Geometry: final body of the model. Coordinates: model frame, mm. Give positions to 0.01 mm unless a question says otherwise; leave off trailing zeros. Loops run counter-clockwise (first coordinate to the right, second up) from the corner with the lowest first, then second, coordinate; pieces in that order, holes last. Notation, with made-up numbers: M 2.5,35 L 34.5,35 A16 ccw 34.5,52 Z; hole C 31,-2.5 d10. An arc over 180 degrees is marked long. One line per question, with ' | ' between items. Start each with the question number.
from build123d import *

# Parameters (mm, degrees)
F0_W        = 105
F0_H        = 20.7723644742
F1_DEPTH    = 3
F2_T1_DEPTH = 58


# Not quite as in the source:
# - a fillet or chamfer that OpenCascade refuses, or shapes differently, is made with other operations: its cross-section is extruded or revolved along the edge and cut away or added


with BuildPart() as f1:
    # F0 (on Front) → F1 (new body)
    with BuildSketch(Plane.XZ):
        Rectangle(F0_W, F0_H)
    extrude(amount=F1_DEPTH)

    # F2: fillet of radius 11 on 4 edges, made by hand

    # F2_s2 → F2_t1 (cut)
    with BuildSketch(Plane.XZ.offset(-27.5)):
        with BuildLine():
            ThreePointArc((-41.5, 10.3861822371), (-49.2781745931, 7.1643568302), (-52.5, -0.6138177629))
            Line((-52.5, -0.6138177629), (-52.5, 10.3861822371))
            Line((-52.5, 10.3861822371), (-41.5, 10.3861822371))
        make_face()
        with BuildLine():
            ThreePointArc((-52.5, 0.6138177629), (-49.2781745931, -7.1643568302), (-41.5, -10.3861822371))
            Line((-41.5, -10.3861822371), (-52.5, -10.3861822371))
            Line((-52.5, -10.3861822371), (-52.5, 0.6138177629))
        make_face()
        with BuildLine():
            ThreePointArc((52.5, -0.6138177629), (49.2781745931, 7.1643568302), (41.5, 10.3861822371))
            Line((41.5, 10.3861822371), (52.5, 10.3861822371))
            Line((52.5, 10.3861822371), (52.5, -0.6138177629))
        make_face()
        with BuildLine():
            ThreePointArc((52.5, 0.6138177629), (49.2781745931, -7.1643568302), (41.5, -10.3861822371))
            Line((41.5, -10.3861822371), (52.5, -10.3861822371))
            Line((52.5, -10.3861822371), (52.5, 0.6138177629))
        make_face()
    extrude(amount=F2_T1_DEPTH, mode=Mode.SUBTRACT)


solid = f1.part
Q1. Material intervals for L1, parallel to X at y = -1.6, z = -0.25; L2, parallel to X at y = -0.6, z = -2; L3, parallel to Z at x = -45, y = -2.1, sorted ascending.
Q2. Section B-B, the plane z = 4. Output: boundary loops of the cut face in (x, y), plus the area to 3 significant figures.
Q3. Contact query for flat-ended pins moving along their axis: pin 1 (1 mm diameter, centred on y = -0.5, z = -5.5, fed in from -X); pin 2 (1 mm diameter, centred on y = -0.5, z = -7, fed in from -X). Output: stop coordinate, or through.
Q4. Section A-A, the plane y = -0.9. Output: boundary loops of the cut face in (x, z).
Q5. Section C-C, the plane x = 46. Output: boundary loops of the cut face in (y, z), plus the area to 3 significant figures.
Model answer:
1) L1: x = -52.47 to 52.47 | L2: x = -52.18 to 52.18 | L3: z = -9.81 to 9.81
2) outline: M -51.49,-3 L 51.49,-3 L 51.49,0 L -51.49,0 Z | area: 309 mm^2
3) pin 1: stops at x = -50.96 | pin 2: stops at x = -49.89
4) outline: M -52.48,0 A11 ccw -41.5,-10.39 L 41.5,-10.39 A11 ccw 52.48,0 A11 ccw 41.5,10.39 L -41.5,10.39 A11 ccw Z
5) outline: M -3,-9.42 L 0,-9.42 L 0,9.42 L -3,9.42 Z | area: 56.5 mm^2
